Could you check a few things on this model? Use its own coordinates, in mm. A direction names the side the tool comes from. Round coordinates to 2 decimals unless told otherwise and drop trailing zeros. Write each loop counter-clockwise with the first axis right and the second up, starting at its lowest first coordinate (ties: lowest second). Pieces come first, ordered by that corner, then holes. Notation, with made-up numbers: M 60.25,-17.5 L 103.25,-17.5 A19 ccw 103.25,11.5 Z; hole C -26.5,10 d7. An arc over 180 degrees is marked long. One line per item, written item: value. Start each with the question number.
(1) Which directions (+Z, -Z, +X, -X, +Y, -Y) give clear straight access to the entire face, cutting with the end or side of a thin tool? Please do faces 4 (the face through (0, 0, 7.5)), 5 (the face through (0, 0, 52.033)), 6 (the face through (11.012, -3.468, 1.893)).
(2) I'm going to push flat-ended pins straight in: pin 1 Ø1 at (y, z) = (-15, 10) entering from +X; pin 2 Ø4 at (x, y) = (-1, -0.5) entering from +Z; pin 3 Ø1.5 at (x, y) = (7.57, 0) entering from +Z; pin 4 Ø2 at (y, z) = (1, 36.5) entering from -X. Where does each tip first touch, or does it pass through?
(3) I want a section at A-A on y = 0. Count the separate pieces of the cut face and the enclosed holes in it, and give its area (3 significant figures).
(4) I want a section at C-C on z = 31. Please give me the cut outline in (x, y).
(5) Thinking about a two-plate mould opening in X: for faces 1 (the face through (-2.53, 11.392, -1.938)), 2 (the face through (-8.803, -0.162, 52.849)), 3 (the face through (9, 9, 9.088)), which applies, released by +X, released by -X, zero draft, split by the parting line, or undercut?
(6) If I drill on L1, parallel to Y at x = 0, z = 53.65; L2, parallel to Y at x = 0, z = 52; L3, parallel to Z at x = 9, y = 4, over which ranges is the centre line in solid material (lowest first)?
```python
from build123d import *

# Parameters (mm, degrees)
ESQUISSE1_R                  = 20
BOSS_EXTRU_1_DEPTH           = 7.5
CONG_1_R                     = 1.7
CONG_3_R                     = 1.7
ESQUISSE5_R                  = 5
ENL_V_MAT_EXTRU_1_DEPTH      = 33.015621312
ESQUISSE8_R                  = 2.54
BOSS_EXTRU_3_DEPTH           = 43.7388
BOSS_EXTRU_4_START           = 1.5875
ESQUISSE9_R                  = 20
BOSS_EXTRU_4_DEPTH           = 1.5875
ESQUISSE10_R                 = 10.2616
BOSS_EXTRU_5_DEPTH           = 3.175
ENL_V_MAT_EXTRU_3_REACH      = 70.068
ESQUISSE11_R                 = 1.2446
R_P_TITION_CIRCULAIRE2_COUNT = 4
ESQUISSE12_R                 = 4.0386
ENL_V_MAT_EXTRU_4_DEPTH      = 2.38125
CHAMFER1_SIZE                = 10
FILLET1_R                    = 10.16


with BuildPart() as part:
    # Esquisse1 → Boss.-Extru.1 (new, symmetric)
    with BuildSketch(Plane.XY):
        Circle(ESQUISSE1_R)
    extrude(amount=BOSS_EXTRU_1_DEPTH, both=True)

    # Esquisse4 → Enlèvement de matière-Révolution1 (revolve, cut)
    with BuildSketch(Plane(origin=(0, 0, 0), x_dir=(0, 0, -1), z_dir=(1, 0, 0)), mode=Mode.PRIVATE) as enl_vement_de_mati_re_r_volution1_sk:
        Polygon((-5, 20), (-1.324936438, 10), (1.324936438, 10), (5, 20), align=None)
    revolve(enl_vement_de_mati_re_r_volution1_sk.sketch.rotate(Axis((0, 0, 15.788572615), (0, 0, -1)), 90), axis=Axis((0, 0, 15.788572615), (0, 0, -1)), mode=Mode.SUBTRACT)

    # Congé1
    cong_1_edges = [part.edges().sort_by_distance(p)[0] for p in [
        (-10, 0, -1.324936438),
    ]]
    fillet(cong_1_edges, radius=CONG_1_R)

    # Congé3
    cong_3_edges = [part.edges().sort_by_distance(p)[0] for p in [
        (-10, 0, 1.324936438),
    ]]
    fillet(cong_3_edges, radius=CONG_3_R)

    # Esquisse5 → Enlèv. mat.-Extru.1 (cut, through all)
    with BuildSketch(Plane.XY.offset(7.5)):
        Circle(ESQUISSE5_R)
    extrude(amount=-ENL_V_MAT_EXTRU_1_DEPTH, mode=Mode.SUBTRACT)



with BuildPart() as body_2:
    # Esquisse8 → Boss.-Extru.3 (new body)
    with BuildSketch(Plane.XY.offset(7.5)):
        Circle(ESQUISSE8_R)
    extrude(amount=BOSS_EXTRU_3_DEPTH)


with BuildPart() as part_1:
    add(part.part)

    add(body_2.part)  # Boss.-Extru.4 merges body 2
    # Esquisse9 → Boss.-Extru.4 (add)
    with BuildSketch(Plane.XY.offset(7.5).offset(BOSS_EXTRU_4_START)):
        Circle(ESQUISSE9_R)
    extrude(amount=-BOSS_EXTRU_4_DEPTH)

    # Esquisse10 → Boss.-Extru.5 (add)
    with BuildSketch(Plane.XY.offset(51.2388)):
        Circle(ESQUISSE10_R)
    extrude(amount=BOSS_EXTRU_5_DEPTH)

    # Esquisse11 → Enlèv. mat.-Extru.3 (cut, up to next)
    with BuildSketch(Plane.XY.offset(54.4138), mode=Mode.PRIVATE) as enl_v_mat_extru_3_sk1:
        with Locations((0, 7.5692)):
            Circle(ESQUISSE11_R)
    enl_v_mat_extru_3_tool1 = extrude(enl_v_mat_extru_3_sk1.sketch, amount=-ENL_V_MAT_EXTRU_3_REACH, mode=Mode.PRIVATE) & part_1.part
    enl_v_mat_extru_3 = enl_v_mat_extru_3_tool1.solids().sort_by_distance((0, 7.5692, 54.4138))[0]
    add(enl_v_mat_extru_3, mode=Mode.SUBTRACT)

    # Répétition circulaire2: Enlèv. mat.-Extru.3 ×4 about axis
    r_p_tition_circulaire2_axis = Axis((0, 0, 0), (0, 0, 1))
    for i in range(1, R_P_TITION_CIRCULAIRE2_COUNT):
        add(enl_v_mat_extru_3.rotate(r_p_tition_circulaire2_axis, i * 360 / R_P_TITION_CIRCULAIRE2_COUNT), mode=Mode.SUBTRACT)

    # Esquisse12 → Enlèv. mat.-Extru.4 (cut)
    with BuildSketch(Plane.XY.offset(54.4138)):
        Circle(ESQUISSE12_R)
    extrude(amount=-ENL_V_MAT_EXTRU_4_DEPTH, mode=Mode.SUBTRACT)

    # Chamfer1
    chamfer1_edges = [part_1.edges().sort_by_distance(p)[0] for p in [
        (-2.54, 0, 9.0875),
    ]]
    chamfer(chamfer1_edges, length=CHAMFER1_SIZE)

    # Fillet1
    fillet1_edges = [part_1.edges().sort_by_distance(p)[0] for p in [
        (-2.54, 0, 19.0875),
    ]]
    fillet(fillet1_edges, radius=FILLET1_R)


solid = part_1.part
```
Found:
1. face 4: -Z
1. face 5: +Z
1. face 6: none
2. pin 1: passes through
2. pin 2: stops at z = 52.03
2. pin 3: stops at z = 14.81
2. pin 4: stops at x = -2.54
3. separate pieces: 3
3. enclosed holes: 0
3. area: 737 mm²
4. outline: C 0,0 d5.08
5. face 1: split by the parting line
5. face 2: undercut
5. face 3: zero draft
6. L1: y = -10.26 to -8.81, -6.32 to -4.04, 4.04 to 6.32, 8.81 to 10.26
6. L2: y = -10.26 to -8.81, -6.32 to 6.32, 8.81 to 10.26
6. L3: z = -7.5 to 11.78, 51.24 to 54.41
